Geometry check sheet. Reference: the model listing, model coordinates, mm. Coordinates: 2 decimals unless noted, no trailing zeros. Order: outer loops, then holes, each group sorted by start corner. A loop starts at its lowest first (then second) coordinate and runs counter-clockwise, first axis right, second up. Notation, with made-up numbers: (5, 53.25) - (28, 53.25) arc R20 cw to (28, 72.25) - close; hole circle Ø9 at (-39.75, -6). An arc over 180 degrees is marked (long way). Use CSV: the item, a comma, the result in double quotes. Start each with the question number.
1) Thickness scan on probe 1 along X at (y, z) = (17, -6); probe 2 along X at (y, z) = (20, 12); probe 3 along Z at (x, y) = (11.5, 18.5). Record the ranges inside material, lowest first. Write a range as [from, to].
2) Sectioned sample at C-C, the plane z = 12.7. Record the cut outline in (x, y) (3 decimals), and give its area (3 significant figures).
3) Sectioned sample at B-B, the plane x = 0. Record the cut outline in (y, z) (3 decimals).
4) Depth check by flat-ended pin: P1, Ø1.5, axis at x = -0.5, z = 13, coming from the +Y side; P2, Ø3, axis at x = 1.5, y = 3, coming from the +Z side (3 decimals); P3, Ø5, axis at y = 20, z = 12, coming from the +X side. Enter the tip coordinate at first touch or a pass-through.
5) Sectioned sample at D-D, the plane y = 10. Record the cut outline in (x, z) (3 decimals).
6) Sectioned sample at A-A, the plane y = 20. Record the cut outline in (x, z) (3 decimals).
from build123d import *

# Parameters (mm, degrees)
SKETCH1_R           = 18.415
BOSS_EXTRUDE1_DEPTH = 25.4
SKETCH2_R           = 1.5
CUT_EXTRUDE1_DEPTH  = 12.7
CIRPATTERN1_COUNT   = 6


with BuildPart() as part:
    # Sketch1 → Boss-Extrude1 (new body, symmetric)
    with BuildSketch(Plane(origin=(0, 0, 0), x_dir=(1, 0, 0), z_dir=(0, 1, 0))):
        Circle(SKETCH1_R)
    extrude(amount=BOSS_EXTRUDE1_DEPTH, both=True)

    # Sketch2 → Cut-Extrude1 (cut)
    with BuildSketch(Plane(origin=(0, 25.4, 0), x_dir=(1, 0, 0), z_dir=(0, 1, 0))):
        with Locations((0, 12.7)):
            Circle(SKETCH2_R)
    cut_extrude1 = extrude(amount=-CUT_EXTRUDE1_DEPTH, mode=Mode.SUBTRACT)

    # CirPattern1: Cut-Extrude1 ×6 about axis
    cirpattern1_axis = Axis((0, 0, 0), (0, 1, 0))
    for i in range(1, CIRPATTERN1_COUNT):
        add(cut_extrude1.rotate(cirpattern1_axis, i * 360 / CIRPATTERN1_COUNT), mode=Mode.SUBTRACT)


solid = part.part
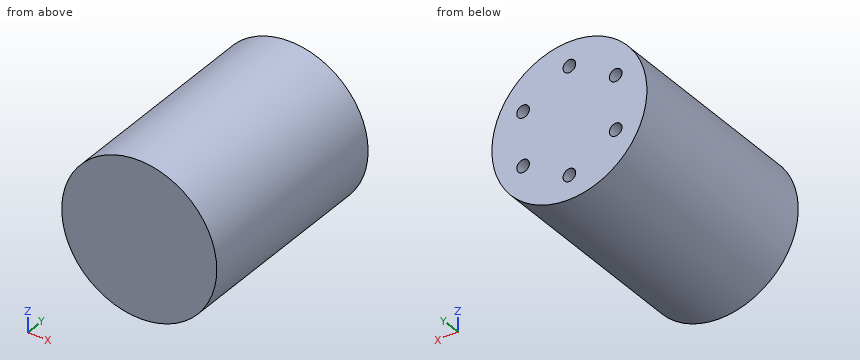
Evaluation:
1,probe 1,"[-17.41, -12.46], [-9.54, 9.54], [12.46, 17.41]"
1,probe 2,"[-13.97, -1.33], [1.33, 13.97]"
1,probe 3,"[-14.38, -7.76], [-4.94, 4.94], [7.76, 14.38]"
2,outline,"(-13.335, -25.4) - (13.335, -25.4) - (13.335, 25.4) - (1.5, 25.4) - (1.5, 12.7) - (-1.5, 12.7) - (-1.5, 25.4) - (-13.335, 25.4) - close"
2,area,"1,320 mm²"
3,outline,"(-25.4, -18.415) - (25.4, -18.415) - (25.4, -14.2) - (12.7, -14.2) - (12.7, -11.2) - (25.4, -11.2) - (25.4, 11.2) - (12.7, 11.2) - (12.7, 14.2) - (25.4, 14.2) - (25.4, 18.415) - (-25.4, 18.415) - close"
4,P1,"y = 12.7"
4,P2,"z = 18.415"
4,P3,"x = 15.78"
5,outline,"circle Ø36.83 at (0, 0)"
6,outline,"circle Ø36.83 at (0, 0); hole circle Ø3 at (-10.999, -6.35); hole circle Ø3 at (-10.999, 6.35); hole circle Ø3 at (0, -12.7); hole circle Ø3 at (0, 12.7); hole circle Ø3 at (10.999, -6.35); hole circle Ø3 at (10.999, 6.35)"
